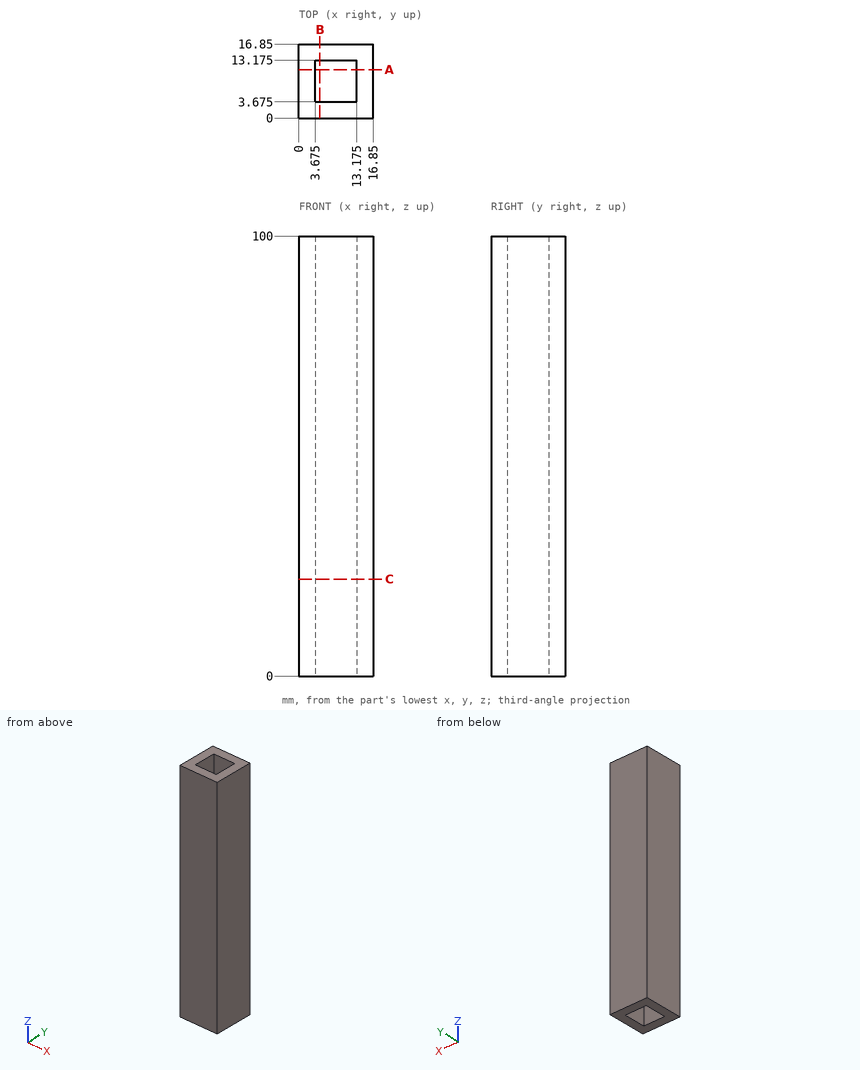
Geometry: see drawing. Coordinates: mm, zero at the bounding-box minimum. Give positions to 0.01 mm unless a question says otherwise; leave off trailing zeros. Order: outer loops, then holes, each group sorted by start corner. A loop starts at its lowest first (then second) coordinate and runs counter-clockwise, first axis right, second up. Notation, with made-up numbers: (62, 75) - (101, 75) arc R25 ccw to (101, 93) - close; hole circle Ø7 at (-16, -4.5). An arc over 180 degrees is marked (long way). Write each question's results on one line, items separated by ' | '.
Item 1: Material intervals for line 1 along X through (y, z) = (11, 8) (3 decimals), sorted ascending.
A:
line 1: x = 0 to 3.675, 13.175 to 16.85
Item 2: Section A-A (y = 11). Return loops of the section in (x, z) (3 decimals), and give its area (3 significant figures).
A:
outline: (0, 0) - (3.675, 0) - (3.675, 100) - (0, 100) - close; (13.175, 0) - (16.85, 0) - (16.85, 100) - (13.175, 100) - close | area: 735 mm^2
Item 3: Contact query for flat-ended pins moving along their axis: pin 1 Ø5 at (x, z) = (6.5, 78.5) entering from -Y; pin 2 Ø2 at (x, y) = (9, 12) entering from +Z. Output: stop coordinate, or through.
A:
pin 1: stops at y = 0 | pin 2: passes through
Item 4: Section C-C (z = 22). Return loops of the section in (x, y) (3 decimals), and give its area (3 significant figures).
A:
outline: (0, 0) - (16.85, 0) - (16.85, 16.85) - (0, 16.85) - close; hole (3.675, 3.675) - (13.175, 3.675) - (13.175, 13.175) - (3.675, 13.175) - close | area: 194 mm^2
